Model file for the job. Use its own axes, mm. Round coordinates to 2 decimals unless told otherwise and drop trailing zeros. Loops run counter-clockwise (first coordinate to the right, second up) from the corner with the lowest first, then second, coordinate; pieces in that order, holes last. Notation, with made-up numbers: (24.25, 58.5) - (38.25, 58.5) arc R16 cw to (38.25, 67.5) - close; hole circle Ø4 at (67, 7). An arc over 180 degrees is marked (long way). Use one line per item in the form item = value.
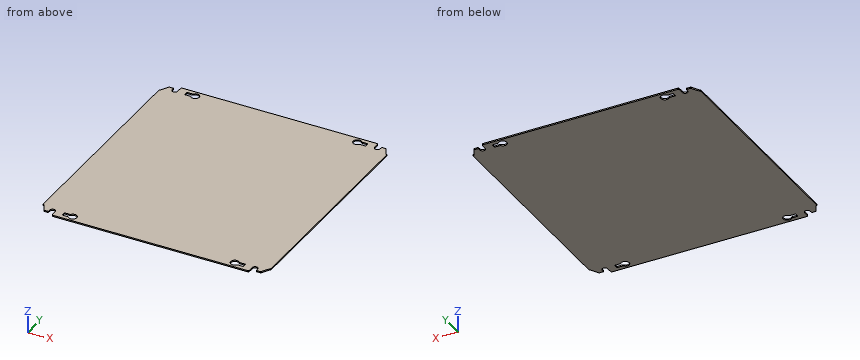
Autodesk Inventor part; units mm, degrees
ref_plane "MP_XY" through (0, 0, 0) normal (0, 0, 1) x (1, 0, 0)
ref_plane "MP_YZ" through (0, 0, 0) normal (1, 0, 0) x (0, 1, 0)
ref_plane "MP_ZX" through (0, 0, 0) normal (0, 1, 0) x (0, 0, 1)
sketch "Sketch_11" plane through (0, 0, 0) normal (0, 0, 1) x (1, 0, 0)
  line L0 (-225, 438.5) -> (-225, 11.5)
  line L1 (-225, 11.5) -> (-224.0774, 11.5)
  arc A0 (-223.2113, 11) -> (-224.0774, 11.5) centre (-224.0774, 10.5) ccw
  line L2 (-223.2113, 11) -> (-214.2624, -4.5)
  arc A1 (-214.2624, -4.5) -> (-213.3964, -5) centre (-213.3964, -4) ccw
  line L3 (-213.3964, -5) -> (-206.5, -5)
  arc A2 (-206.5, -5) -> (-205.5, -4) centre (-206.5, -4) ccw
  line L4 (-205.5, -4) -> (-205.5, 0)
  arc A3 (-194.5, 0) -> (-205.5, 0) centre (-200, 0) ccw
  line L5 (-194.5, 0) -> (-194.5, -11)
  line L6 (-194.5, -11) -> (-193, -12.5)
  line L7 (-193, -12.5) -> (193, -12.5)
  line L8 (193, -12.5) -> (194.5, -11)
  line L9 (194.5, -11) -> (194.5, 0)
  arc A4 (205.5, 0) -> (194.5, 0) centre (200, 0) ccw
  line L10 (205.5, 0) -> (205.5, -4)
  arc A5 (205.5, -4) -> (206.5, -5) centre (206.5, -4) ccw
  line L11 (206.5, -5) -> (213.3964, -5)
  arc A6 (213.3964, -5) -> (214.2624, -4.5) centre (213.3964, -4) ccw
  line L12 (214.2624, -4.5) -> (223.2113, 11)
  arc A7 (224.0774, 11.5) -> (223.2113, 11) centre (224.0774, 10.5) ccw
  line L13 (224.0774, 11.5) -> (225, 11.5)
  line L14 (225, 11.5) -> (225, 438.5)
  line L15 (225, 438.5) -> (224.0774, 438.5)
  arc A8 (223.2113, 439) -> (224.0774, 438.5) centre (224.0774, 439.5) ccw
  line L16 (223.2113, 439) -> (214.2624, 454.5)
  arc A9 (214.2624, 454.5) -> (213.3964, 455) centre (213.3964, 454) ccw
  line L17 (213.3964, 455) -> (206.5, 455)
  arc A10 (206.5, 455) -> (205.5, 454) centre (206.5, 454) ccw
  line L18 (205.5, 454) -> (205.5, 450)
  arc A11 (194.5, 450) -> (205.5, 450) centre (200, 450) ccw
  line L19 (194.5, 450) -> (194.5, 461)
  line L20 (194.5, 461) -> (193, 462.5)
  line L21 (193, 462.5) -> (-193, 462.5)
  line L22 (-193, 462.5) -> (-194.5, 461)
  line L23 (-194.5, 461) -> (-194.5, 450)
  arc A12 (-205.5, 450) -> (-194.5, 450) centre (-200, 450) ccw
  line L24 (-205.5, 450) -> (-205.5, 454)
  arc A13 (-205.5, 454) -> (-206.5, 455) centre (-206.5, 454) ccw
  line L25 (-206.5, 455) -> (-213.3964, 455)
  arc A14 (-213.3964, 455) -> (-214.2624, 454.5) centre (-213.3964, 454) ccw
  line L26 (-214.2624, 454.5) -> (-223.2113, 439)
  arc A15 (-224.0774, 438.5) -> (-223.2113, 439) centre (-224.0774, 439.5) ccw
  line L27 (-224.0774, 438.5) -> (-225, 438.5)
  arc A16 (166.5296, 4.6222) -> (166.5296, -4.6222) centre (160, 0) ccw
  arc A17 (167.3457, -4.2) -> (166.5296, -4.6222) centre (167.3457, -5.2) ccw
  line L28 (167.3457, -4.2) -> (178, -4.2)
  arc A18 (178, -4.2) -> (179, -3.2) centre (178, -3.2) ccw
  line L29 (179, -3.2) -> (179, 3.2)
  arc A19 (179, 3.2) -> (178, 4.2) centre (178, 3.2) ccw
  line L30 (178, 4.2) -> (167.3457, 4.2)
  arc A20 (166.5296, 4.6222) -> (167.3457, 4.2) centre (167.3457, 5.2) ccw
  arc A21 (166.5296, 454.6222) -> (166.5296, 445.3778) centre (160, 450) ccw
  arc A22 (167.3457, 445.8) -> (166.5296, 445.3778) centre (167.3457, 444.8) ccw
  line L31 (167.3457, 445.8) -> (178, 445.8)
  arc A23 (178, 445.8) -> (179, 446.8) centre (178, 446.8) ccw
  line L32 (179, 446.8) -> (179, 453.2)
  arc A24 (179, 453.2) -> (178, 454.2) centre (178, 453.2) ccw
  line L33 (178, 454.2) -> (167.3457, 454.2)
  arc A25 (166.5296, 454.6222) -> (167.3457, 454.2) centre (167.3457, 455.2) ccw
  line L34 (-179, 3.2) -> (-179, -3.2)
  arc A26 (-179, -3.2) -> (-178, -4.2) centre (-178, -3.2) ccw
  line L35 (-178, -4.2) -> (-167.3457, -4.2)
  arc A27 (-166.5296, -4.6222) -> (-167.3457, -4.2) centre (-167.3457, -5.2) ccw
  arc A28 (-166.5296, -4.6222) -> (-166.5296, 4.6222) centre (-160, 0) ccw
  arc A29 (-167.3457, 4.2) -> (-166.5296, 4.6222) centre (-167.3457, 5.2) ccw
  line L36 (-167.3457, 4.2) -> (-178, 4.2)
  arc A30 (-178, 4.2) -> (-179, 3.2) centre (-178, 3.2) ccw
  arc A31 (-179, 446.8) -> (-178, 445.8) centre (-178, 446.8) ccw
  line L37 (-178, 445.8) -> (-167.3457, 445.8)
  arc A32 (-166.5296, 445.3778) -> (-167.3457, 445.8) centre (-167.3457, 444.8) ccw
  arc A33 (-166.5296, 445.3778) -> (-166.5296, 454.6222) centre (-160, 450) ccw
  arc A34 (-167.3457, 454.2) -> (-166.5296, 454.6222) centre (-167.3457, 455.2) ccw
  line L38 (-167.3457, 454.2) -> (-178, 454.2)
  arc A35 (-178, 454.2) -> (-179, 453.2) centre (-178, 453.2) ccw
  line L39 (-179, 453.2) -> (-179, 446.8)
extrude "Extrusion1" add sketch "Sketch_11" against normal blind 2.5
ref_plane "MP_XY" through (0, 0, 0) normal (0, 0, 1) x (1, 0, 0)
ref_plane "MP_YZ" through (0, 0, 0) normal (1, 0, 0) x (0, 1, 0)
ref_plane "MP_ZX" through (0, 0, 0) normal (0, 1, 0) x (0, 0, 1)
ref_plane "to_EB_XY" through (174.8, 0, -2.5) normal (0, 0, 1) x (1, 0, 0)
ref_plane "to_EB_YZ" through (174.8, 0, -2.5) normal (1, 0, 0) x (0, 1, 0)
ref_plane "to_EB_ZX" through (174.8, 0, -2.5) normal (0, 1, 0) x (0, 0, 1)
properties part number "155X_02_00_P6_(1)"
1. Cut at B-B, the plane x = -200. Give the cut face in (y, z), plus the area to 3 significant figures.
Geometry check:
outline = (5.5, -2.5) - (444.5, -2.5) - (444.5, 0) - (5.5, 0) - close
area = 1,100 mm^2
2. Flat gauge pins, fed straight in: pin 1 (5 mm diameter, centred on x = -83, y = 222, fed in from +Z); pin 2 (1.2 mm diameter, centred on y = 453.5, z = -1.5, fed in from +X); pin 3 (1.2 mm diameter, centred on x = -209, z = -1, fed in from +Y); pin 4 (0.5 mm diameter, centred on x = 224.5, z = -1.5, fed in from -Y). Where does each tip first touch, or does it go through?
Geometry check:
pin_1 = 0
pin_2 = 215.19
pin_3 = 455
pin_4 = 11.5
3. Cut at A-A, the plane x = 160. Give the cut face in (y, z).
Geometry check:
outline = (-12.5, -2.5) - (-8, -2.5) - (-8, 0) - (-12.5, 0) - close; (8, -2.5) - (442, -2.5) - (442, 0) - (8, 0) - close; (458, -2.5) - (462.5, -2.5) - (462.5, 0) - (458, 0) - close
4. Wall check: probe 1 along Y at (x, z) = (160, -1.95); probe 2 along Y at (x, z) = (-154.5, -0.75); probe 3 along X at (y, z) = (450, -1.3). Give the ranges that are in metal, low to high.
Geometry check:
probe_1 = -12.5 to -8, 8 to 442, 458 to 462.5
probe_2 = -12.5 to -5.81, 5.81 to 444.19, 455.81 to 462.5
probe_3 = -216.86 to -205.5, -194.5 to -179, -152 to 152, 179 to 194.5, 205.5 to 216.86
